CAD build for the part. Positions are in the model's coordinates, mm. A direction names the side the tool comes from. Give positions to 0.01 mm unless a question says otherwise; leave off trailing zeros. Loops run counter-clockwise (first coordinate to the right, second up) from the corner with the lowest first, then second, coordinate; pieces in that order, holes last. Notation, with made-up numbers: (12, 51.5) - (36, 51.5) arc R19 cw to (36, 75.5) - close; hole circle Ø8 at (38, -21). An arc over 180 degrees is marked (long way). Return JSON: item names as keys, results as strings.
from build123d import *

# Parameters (mm, degrees)
SKETCH3_R           = 2
BOSS_EXTRUDE1_DEPTH = 2
SKETCH4_W           = 25
SKETCH4_H           = 2
BOSS_EXTRUDE2_DEPTH = 25
CUT_EXTRUDE1_REACH  = 58.578
SKETCH6_R           = 1
FILLET1_R           = 2


with BuildPart() as part:
    # Sketch3 → Boss-Extrude1 (new body)
    with BuildSketch(Plane(origin=(0, 0, 0), x_dir=(1, 0, 0), z_dir=(0, 1, 0))):
        with BuildLine():
            ThreePointArc((8.728627884, 6), (8.109373095, 2.770911469), (6.339475115, 0))
            ThreePointArc((6.339475115, 0), (0, -2.728627884), (-6.339475115, 0))
            ThreePointArc((-6.339475115, 0), (-8.109373095, 2.770911469), (-8.728627884, 6))
            Line((-8.728627884, 6), (-48.25, 6))
            Line((-48.25, 6), (-48.25, -6))
            Line((-48.25, -6), (48.25, -6))
            Line((48.25, -6), (48.25, 6))
            Line((48.25, 6), (8.728627884, 6))
        make_face()
        with Locations(Location((-42.25, 0, 0), (0, 0, 270))):
            Circle(SKETCH3_R, mode=Mode.SUBTRACT)
        with BuildLine():
            ThreePointArc((44.25, 0), (42.25, -2), (40.25, 0))
            ThreePointArc((40.25, 0), (42.25, 2), (44.25, 0))
        make_face(mode=Mode.SUBTRACT)
    extrude(amount=BOSS_EXTRUDE1_DEPTH)

    # Sketch4 → Boss-Extrude2 (add)
    with BuildSketch(Plane(origin=(0, 2, 0), x_dir=(1, 0, 0), z_dir=(0, 1, 0))):
        with Locations((-12.5, -5)):
            Rectangle(SKETCH4_W, SKETCH4_H)
        with Locations((12.5, -5)):
            Rectangle(SKETCH4_W, SKETCH4_H)
    extrude(amount=BOSS_EXTRUDE2_DEPTH)

    # Sketch6 → Cut-Extrude1 (cut, up to next)
    with BuildSketch(Plane.XY.offset(6), mode=Mode.PRIVATE) as cut_extrude1_sk1:
        with Locations((21.25, 23.354759591)):
            Circle(SKETCH6_R)
    cut_extrude1_tool1 = extrude(cut_extrude1_sk1.sketch, amount=-CUT_EXTRUDE1_REACH, mode=Mode.PRIVATE) & part.part
    # Sketch6 → Cut-Extrude1 (cut, up to next)
    with BuildSketch(Plane.XY.offset(6), mode=Mode.PRIVATE) as cut_extrude1_sk2:
        with Locations((-21.25, 23.354759591)):
            Circle(SKETCH6_R)
    cut_extrude1_tool2 = extrude(cut_extrude1_sk2.sketch, amount=-CUT_EXTRUDE1_REACH, mode=Mode.PRIVATE) & part.part
    # Sketch6 → Cut-Extrude1 (cut, up to next)
    with BuildSketch(Plane.XY.offset(6), mode=Mode.PRIVATE) as cut_extrude1_sk3:
        with Locations((21.25, 6.354759591)):
            Circle(SKETCH6_R)
    cut_extrude1_tool3 = extrude(cut_extrude1_sk3.sketch, amount=-CUT_EXTRUDE1_REACH, mode=Mode.PRIVATE) & part.part
    # Sketch6 → Cut-Extrude1 (cut, up to next)
    with BuildSketch(Plane.XY.offset(6), mode=Mode.PRIVATE) as cut_extrude1_sk4:
        with Locations((-21.25, 6.354759591)):
            Circle(SKETCH6_R)
    cut_extrude1_tool4 = extrude(cut_extrude1_sk4.sketch, amount=-CUT_EXTRUDE1_REACH, mode=Mode.PRIVATE) & part.part
    add(cut_extrude1_tool1.solids().sort_by_distance((21.25, 23.35476, 6))[0], mode=Mode.SUBTRACT)
    add(cut_extrude1_tool2.solids().sort_by_distance((-21.25, 23.35476, 6))[0], mode=Mode.SUBTRACT)
    add(cut_extrude1_tool3.solids().sort_by_distance((21.25, 6.35476, 6))[0], mode=Mode.SUBTRACT)
    add(cut_extrude1_tool4.solids().sort_by_distance((-21.25, 6.35476, 6))[0], mode=Mode.SUBTRACT)

    # Fillet1
    fillet1_edges = [part.edges().sort_by_distance(p)[0] for p in [
        (8.728627884, 1, -6),
        (48.25, 1, -6),
        (48.25, 1, 6),
        (-48.25, 1, 6),
        (-48.25, 1, -6),
        (-8.728627884, 1, -6),
        (25, 27, 5),
        (-25, 27, 5),
    ]]
    fillet(fillet1_edges, radius=FILLET1_R)


solid = part.part
1. Pull direction X, two halves, no side cores. Call faces 1 (the face through (-48.25, 1, 0)), 2 (the face through (-28, 1, -6)), 3 (the face through (-44.202, 0.986, -0.434)), 4 (the face through (25, 13, 5)): +X half, -X half, draft (parallel to the pull), parting line (faces both ways), or undercut.
Values follow:
{"face 1": "-X half", "face 2": "draft", "face 3": "undercut", "face 4": "+X half"}
2. Drill centre lines: probe 1 along Y at (x, z) = (-21.25, 5.25); probe 2 along Z at (x, y) = (2.5, 6.25); probe 3 along Y at (x, z) = (-41, 5.5). Where is each one in solid material? Low to high.
Values follow:
{"probe 1": "y = 0 to 5.35, 7.35 to 22.35, 24.35 to 27", "probe 2": "z = 4 to 6", "probe 3": "y = 0 to 2"}
3. Cut at C-C, the plane x = 37.5. Write the cut outline in (y, z), plus the area to 3 significant figures.
Values follow:
{"outline": "(0, -6) - (2, -6) - (2, 6) - (0, 6) - close", "area": "24.0 mm²"}
4. Cut at A-A, the plane x = -42.25. Write the cut outline in (y, z).
Values follow:
{"outline": "(0, -6) - (2, -6) - (2, -2) - (0, -2) - close; (0, 2) - (2, 2) - (2, 6) - (0, 6) - close"}
5. Drop flat-ended pins along their axis: P1, Ø0.6, axis at y = 17.5, z = 5, coming from the +X side; P2, Ø4.5, axis at x = 42.25, z = 0, coming from the -Y side; P3, Ø2.5, axis at x = -21.25, y = 23.35, coming from the -Z side; P4, Ø2, axis at y = 16, z = 5, coming from the -X side. Give the stop position or say it passes through.
Values follow:
{"P1": "stops at x = 25", "P2": "stops at y = 0", "P3": "stops at z = 4", "P4": "stops at x = -25"}
6. Which spindle directions (+Z, -Z, +X, -X, +Y, -Y) get a long thin tool onto all of the face, cutting with end or side? Do faces 5 (the face through (-9.25, 1.01, -5.53)), 6 (the face through (-47.65, 1.01, 5.43)). Say none if no direction does.
Values follow:
{"face 5": "-Z, +Y, -Y", "face 6": "+Z, -X, +Y, -Y"}
7. Cut at B-B, the plane x = 21.25. Write the cut outline in (y, z), plus the area to 3 significant figures.
Values follow:
{"outline": "(0, -6) - (2, -6) - (2, 4) - (5.35, 4) - (5.35, 6) - (0, 6) - close; (7.35, 4) - (22.35, 4) - (22.35, 6) - (7.35, 6) - close; (24.35, 4) - (27, 4) - (27, 6) - (24.35, 6) - close", "area": "66.0 mm²"}
